Source: CAD feature listing. Evaluate the final solid. Frame: model axes, mm. A direction names the side the tool comes from. Round coordinates to 2 decimals unless told otherwise and drop trailing zeros. Loops run counter-clockwise (first coordinate to the right, second up) from the corner with the lowest first, then second, coordinate; pieces in that order, holes last. Notation, with made-up numbers: (33.5, -1) -> (85.5, -1) arc R26 ccw to (85.5, 29) -> close; hole circle Ø4 at (-11.5, 81.5). An arc over 180 degrees is marked (long way). Return JSON: item names as keys, results as strings. Group by question number.
```python
from build123d import *

# Parameters (mm, degrees)
F1_DEPTH  = 50.8
F3_DEPTH  = 50.8
F4_R      = 3.175
F5_DEPTH  = 50.8
F5_FACE_R = 3.175
F6_DEPTH  = 9.144
F7_W      = 2.072896
F7_H      = 22.642412
F8_DEPTH  = 44.45
F8_FACE_W = 2.072896
F8_FACE_H = 22.642412
F9_DEPTH  = 17.78


with BuildPart() as f1:
    # F0 (on Front) → F1 (new body)
    with BuildSketch(Plane.XZ):
        with BuildLine():
            Line((5.037427, 65.466186), (0, 69.3323))
            ThreePointArc((0, 69.3323), (-24.938895, -4.123856), (0, -77.580011))
            Line((0, -77.580011), (5.037427, -73.713898))
            ThreePointArc((5.037427, -73.713898), (-18.588894, -4.123856), (5.037427, 65.466186))
        make_face()
    extrude(amount=-F1_DEPTH)

    # F2 (on Right) → F3 (cut)
    with BuildSketch(Plane.YZ):
        with BuildLine():
            Line((17.769823, 33.552193), (10.784823, 33.552193))
            ThreePointArc((10.784823, 33.552193), (9.886797, 33.180219), (9.514823, 32.282193))
            Line((9.514823, 32.282193), (9.514823, -35.027807))
            ThreePointArc((9.514823, -35.027807), (9.886797, -35.925833), (10.784823, -36.297807))
            Line((10.784823, -36.297807), (17.769823, -36.297807))
            ThreePointArc((17.769823, -36.297807), (18.667848, -35.925833), (19.039823, -35.027807))
            Line((19.039823, -35.027807), (19.039823, 32.282193))
            ThreePointArc((19.039823, 32.282193), (18.667848, 33.180219), (17.769823, 33.552193))
        make_face()
    extrude(amount=-F3_DEPTH, mode=Mode.SUBTRACT)

    # F4 (on Right) → F5 (join)
    with BuildSketch(Plane.YZ):
        with Locations((32.150656, 45.544412)):
            Circle(F4_R)
        with Locations((30.170465, -45.724433)):
            Circle(F4_R)
    extrude(amount=-F5_DEPTH)

    # F5_face (on face) → F6 (cut)
    with BuildSketch(Plane(origin=(0, 32.150656, 45.544412), x_dir=(0, 1, 0), z_dir=(1, 0, 0))):
        Circle(F5_FACE_R)
        with Locations((-1.980191, -91.268845)):
            Circle(F5_FACE_R)
    extrude(amount=-F6_DEPTH, mode=Mode.SUBTRACT)

    # F7 (on Right) → F8 (join)
    with BuildSketch(Plane.YZ):
        with Locations((6.339868, 0.01599)):
            Rectangle(F7_W, F7_H)
    extrude(amount=-F8_DEPTH)

    # F8_face (on face) → F9 (cut)
    with BuildSketch(Plane(origin=(0, 6.339868, 0.01599), x_dir=(0, 1, 0), z_dir=(1, 0, 0))):
        Rectangle(F8_FACE_W, F8_FACE_H)
    extrude(amount=-F9_DEPTH, mode=Mode.SUBTRACT)


solid = f1.part
```
(1) Ray query, line 1 (Z direction, x = -1, y = 39.5); line 2 (Z direction, x = 0, y = 8.5); line 3 (Y direction, x = -30.5, z = 1). Return the intervals inside material, ascending.
(2) Pin query (flat end, axial travel): pin 1 (16.5 mm diameter, centred on x = -38.5, z = 3, fed in from -Y); pin 2 (1.7 mm diameter, centred on x = -35, y = 6, fed in from -Z); pin 3 (7.5 mm diameter, centred on x = -17, y = 14.5, fed in from -Z). Return the tip coordinate at first contact, or that it passes through.
(3) Cut plane D-D (y = 21.5). Return loops of the section in (x, z), and give its area (3 significant figures).
(4) Cut plane B-B (z = -31.5). Return loops of the section in (x, y).
(5) Cut plane A-A (y = 15.5). Return loops of the section in (x, z).
(6) Cut plane C-C (x = -27). Return loops of the section in (y, z) (3 decimals).
(7) Set-up query: faces 1 (the face through (-20, 19.04, -2)), 2 (the face through (-33.32, 31.64, -48.54)), 3 (the face through (-9.144, 32, 46)), 4 (the face through (-9.144, 30, -46)). Return all of +Z, -Z, +X, -X, +Y, -Y with unobstructed straight access to the full face (end or side cutting, diameter ignored); none if empty.
Answers follow:
{
 "1": {"line 1": "-76.26 to -65.05, 56.8 to 68.01", "line 2": "-77.58 to -66.6, 58.36 to 69.33", "line 3": "5.3 to 7.38"},
 "2": {"pin 1": "y = 5.3", "pin 2": "z = -11.31", "pin 3": "z = -55.93"},
 "3": {"outline": "(0, -77.58) -> (5.04, -73.71) arc R114.3 cw to (5.04, 65.47) -> (0, 69.33) arc R120.65 ccw to start", "area": "977 mm^2"},
 "4": {"outline": "(-21.79, 0) -> (-15.26, 0) -> (-15.26, 9.51) -> (-21.79, 9.51) -> close; (-21.79, 19.04) -> (-15.26, 19.04) -> (-15.26, 50.8) -> (-21.79, 50.8) -> close"},
 "5": {"outline": "(-20.57, -36.3) arc R120.65 ccw to (0, -77.58) -> (5.04, -73.71) arc R114.3 cw to (-13.97, -36.3) -> close; (-18.91, 33.55) -> (-12.2, 33.55) arc R114.3 cw to (5.04, 65.47) -> (0, 69.33) arc R120.65 ccw to start"},
 "6": {"outline": "(5.303, -11.305) -> (7.376, -11.305) -> (7.376, 11.337) -> (5.303, 11.337) -> close; circle Ø6.35 at (30.17, -45.724); circle Ø6.35 at (32.151, 45.544)"},
 "7": {"face 1": "+X, -X", "face 2": "-X", "face 3": "+X", "face 4": "+X, +Y, -Y"}
}
